Verification items for the finished model (mm, model axes). A direction names the side the tool comes from. Give positions to 0.01 mm unless a question says otherwise; leave off trailing zeros. Write each loop counter-clockwise with the first axis right and the second up, starting at its lowest first coordinate (ties: lowest second). Pieces come first, ordered by that corner, then holes.
from build123d import *

# Parameters (mm, degrees)
SKETCH2_W           = 70
SKETCH2_H           = 110
BOSS_EXTRUDE1_DEPTH = 2.5
SKETCH3_W           = 65
SKETCH3_H           = 2.5
BOSS_EXTRUDE2_DEPTH = 5
SKETCH4_W           = 2.5
SKETCH4_H           = 15
BOSS_EXTRUDE3_DEPTH = 15
SKETCH6_R           = 1.6
CUT_EXTRUDE1_DEPTH  = 89.811598342
SKETCH7_W           = 25
SKETCH7_H           = 17
SKETCH7_R           = 5.5
CUT_EXTRUDE2_DEPTH  = 68.5
FILLET1_R           = 2.5
FILLET2_R           = 2.5


with BuildPart() as part:
    # Sketch2 → Boss-Extrude1 (new body)
    with BuildSketch(Plane(origin=(0, 0, 0), x_dir=(1, 0, 0), z_dir=(0, 1, 0))):
        Rectangle(SKETCH2_W, SKETCH2_H)
    extrude(amount=BOSS_EXTRUDE1_DEPTH)

    # Sketch3 → Boss-Extrude2 (add)
    with BuildSketch(Plane(origin=(0, 2.5, 0), x_dir=(1, 0, 0), z_dir=(0, 1, 0))):
        Polygon((-35, 55), (-35, -55), (-32.5, -55), (-32.5, -52.5), (-32.5, 52.5), (-32.5, 55), align=None)
        Polygon((35, 55), (-32.5, 55), (-32.5, 52.5), (32.5, 52.5), (35, 52.5), align=None)
        Polygon((32.5, -52.5), (32.5, -55), (35, -55), (35, 52.5), (32.5, 52.5), align=None)
        with Locations((0, -53.75)):
            Rectangle(SKETCH3_W, SKETCH3_H)
    extrude(amount=BOSS_EXTRUDE2_DEPTH)

    # Sketch4 → Boss-Extrude3 (add)
    with BuildSketch(Plane(origin=(0, 2.5, 0), x_dir=(1, 0, 0), z_dir=(0, 1, 0))):
        with Locations((-31.25, 37.5)):
            Rectangle(SKETCH4_W, SKETCH4_H)
        with Locations((31.25, 37.5)):
            Rectangle(SKETCH4_W, SKETCH4_H)
        with Locations((31.25, -37.5)):
            Rectangle(SKETCH4_W, SKETCH4_H)
        with Locations((-31.25, -37.5)):
            Rectangle(SKETCH4_W, SKETCH4_H)
    extrude(amount=BOSS_EXTRUDE3_DEPTH)

    # Sketch6 → Cut-Extrude1 (cut, through all)
    with BuildSketch(Plane.ZY.offset(32.5)):
        with Locations((-37.5, 12.5)):
            Circle(SKETCH6_R)
        with Locations((37.5, 12.5)):
            Circle(SKETCH6_R)
    extrude(amount=-CUT_EXTRUDE1_DEPTH, mode=Mode.SUBTRACT)

    # Sketch7 → Cut-Extrude2 (cut, through all)
    with BuildSketch(Plane.XZ):
        with Locations((-0.53, 16.5)):
            Rectangle(SKETCH7_W, SKETCH7_H)
        with Locations(Location((0, -22, 0), (0, 0, 270))):
            Circle(SKETCH7_R)
    extrude(amount=-CUT_EXTRUDE2_DEPTH, mode=Mode.SUBTRACT)

    # Fillet1
    fillet1_edges = [part.edges().sort_by_distance(p)[0] for p in [
        (-0.53, 0, 25),
        (11.97, 0, 16.5),
        (-0.53, 0, 8),
        (-13.03, 0, 16.5),
    ]]
    fillet(fillet1_edges, radius=FILLET1_R - 0.0001)  # a hair under: the kernel refuses the full size

    # Fillet2
    fillet2_edges = [part.edges().sort_by_distance(p)[0] for p in [
        (0, 0, -55),
        (35, 0, 0),
        (0, 0, 55),
        (-35, 0, 0),
        (-35, 3.75, -55),
        (35, 3.75, -55),
        (35, 3.75, 55),
        (-35, 3.75, 55),
    ]]
    fillet(fillet2_edges, radius=FILLET2_R)


solid = part.part
Item 1: Set-up check for faces 4 (the face through (31.232, 14.086, 37.292)), 5 (the face through (-31, 10, 45)), 6 (the face through (-0.32, 0.713, 7.248)), 7 (the face through (-34.248, 0.713, -0.735)), 8 (the face through (-32.5, 12.4, -35.7)): record each of +Z, -Z, +X, -X, +Y, -Y from which the full face is reachable in a straight line by a thin tool's end or side.
Answer key:
face 4: +X, -X
face 5: +Y
face 6: -Y
face 7: +Z, -Z, -X, -Y
face 8: +Z, -Z, -X, +Y
Item 2: Scan lines: line 1 along Z through (x, y) = (-31, 7); line 2 along Y through (x, z) = (30.9, -37.5); line 3 along X through (y, z) = (5.25, -2.5). Record each from-to range of solid material in increasing order.
Answer key:
line 1: z = -55 to -52.5, -45 to -30, 30 to 45, 52.5 to 55
line 2: y = 0 to 10.9, 14.1 to 17.5
line 3: x = -35 to -32.5, 32.5 to 35
Item 3: Sectioned sample at C-C on z = 37.5. Record the cut outline in (x, y).
Answer key:
outline: (-35, 2.5) arc R2.5 ccw to (-32.5, 0) - (32.5, 0) arc R2.5 ccw to (35, 2.5) - (35, 7.5) - (32.5, 7.5) - (32.5, 10.9) - (30, 10.9) - (30, 2.5) - (-30, 2.5) - (-30, 10.9) - (-32.5, 10.9) - (-32.5, 7.5) - (-35, 7.5) - close; (-32.5, 14.1) - (-30, 14.1) - (-30, 17.5) - (-32.5, 17.5) - close; (30, 14.1) - (32.5, 14.1) - (32.5, 17.5) - (30, 17.5) - close
Item 4: Sectioned sample at D-D on x = -22.5. Record the cut outline in (y, z).
Answer key:
outline: (0, -52.5) arc R2.5 ccw to (2.5, -55) - (7.5, -55) - (7.5, -52.5) - (2.5, -52.5) - (2.5, 52.5) - (7.5, 52.5) - (7.5, 55) - (2.5, 55) arc R2.5 ccw to (0, 52.5) - close
Item 5: Sectioned sample at A-A on x = 0. State how many separate pieces and enclosed holes the cut face has, then the cut area to 3 significant figures.
Answer key:
separate pieces: 3
enclosed holes: 0
area: 225 mm2
Item 6: Release check for a two-part mould opening along X. For faces 1 (the face through (0.455, 0.713, 54.248)), 2 (the face through (-34.287, 4.965, -54.248)), 3 (the face through (31, 10, 30)) record: released by +X, released by -X, zero draft, split by the parting line, or undercut.
Answer key:
face 1: zero draft
face 2: released by -X
face 3: undercut
Item 7: Depth check by flat-ended pin: pin 1 (6 mm diameter, centred on x = 25, z = -25, fed in from +Y); pin 2 (2 mm diameter, centred on x = 31.5, y = 9, fed in from -Z); pin 3 (10 mm diameter, centred on y = 13, z = 32.5, fed in from -X). Enter the tip coordinate at first touch or a pass-through.
Answer key:
pin 1: stops at y = 2.5
pin 2: stops at z = -45
pin 3: stops at x = -32.5
Item 8: Sectioned sample at B-B on z = -22. Record the cut outline in (x, y).
Answer key:
outline: (-35, 2.5) arc R2.5 ccw to (-32.5, 0) - (-5.5, 0) - (-5.5, 2.5) - (-32.5, 2.5) - (-32.5, 7.5) - (-35, 7.5) - close; (5.5, 0) - (32.5, 0) arc R2.5 ccw to (35, 2.5) - (35, 7.5) - (32.5, 7.5) - (32.5, 2.5) - (5.5, 2.5) - close
